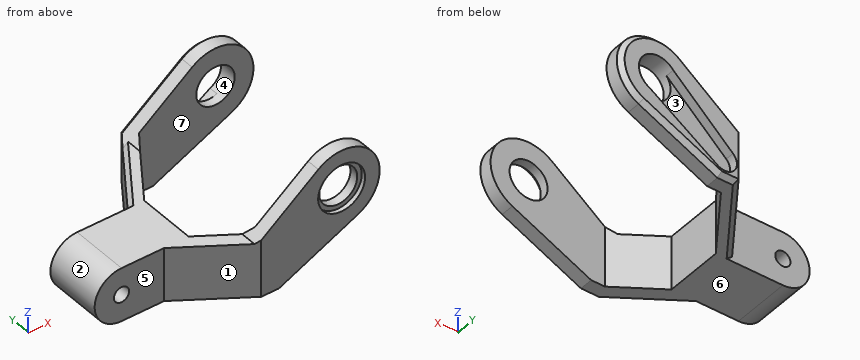
```python
from build123d import *

# Parameters (mm, degrees)
PAD012_DEPTH           = 10
CYLINDER024_R          = 4.3
CYLINDER024_DEPTH      = 14
CYLINDER024_ROLL_ANGLE = 90
CYLINDER017_R          = 4.25
CYLINDER017_DEPTH      = 10
CYLINDER016_R          = 5.25
CYLINDER016_DEPTH      = 10
FUSION009_ROLL_ANGLE   = 90
SKETCH005_R            = 1.7
PAD005_DEPTH           = 50
PAD006_DEPTH           = 40
CHAMFER004_SIZE        = 1


with BuildPart() as pad012:
    # Sketch012 → Pad012 (new body)
    with BuildSketch(Plane(origin=(0, 49, 0), x_dir=(-1, 0, 0), z_dir=(0, 1, 0))):
        with BuildLine():
            ThreePointArc((49.900014, 10.106834), (43.673915, 9.645687), (44.625156, 3.475427))
            Line((44.625156, 3.475427), (60.33289, -7.108383))
            ThreePointArc((60.33289, -7.108383), (64.021726, -6.539695), (63.746037, -2.817476))
            Line((49.900014, 10.106834), (63.746037, -2.817476))
        make_face()
    extrude(amount=PAD012_DEPTH)


with BuildPart() as fusion025:
    # Cylinder024 → Cylinder024 (new body)
    with BuildSketch(Plane.XY):
        Circle(CYLINDER024_R)
    extrude(amount=CYLINDER024_DEPTH)


with BuildPart() as fusion025_1:
    # Cylinder024 roll: moved
    add(fusion025.part.rotate(Axis((0, 0, 0), (1, 0, 0)), CYLINDER024_ROLL_ANGLE))


with BuildPart() as fusion025_2:
    # Cylinder024 placement: moved
    add(fusion025_1.part.moved(Location((-47, 58, 7))))

    # Fusion025: union Pad012
    add(pad012.part)


with BuildPart() as cylinder017:
    # Cylinder017 → Cylinder017 (new body)
    with BuildSketch(Plane.XY.offset(-5)):
        Circle(CYLINDER017_R)
    extrude(amount=CYLINDER017_DEPTH)


with BuildPart() as fusion009:
    # Cylinder016 → Cylinder016 (new body)
    with BuildSketch(Plane.XY):
        Circle(CYLINDER016_R)
    extrude(amount=CYLINDER016_DEPTH)

    # Fusion009: union Cylinder017
    add(cylinder017.part)


with BuildPart() as fusion009_1:
    # Fusion009 roll: moved
    add(fusion009.part.rotate(Axis((0, 0, 0), (1, 0, 0)), FUSION009_ROLL_ANGLE))


with BuildPart() as fusion009_2:
    # Fusion009 placement: moved
    add(fusion009_1.part.moved(Location((-47, 11, 7))))


with BuildPart() as pad005:
    # Sketch005 → Pad005 (new body)
    with BuildSketch(Plane(origin=(0, 55, 0), x_dir=(-1, 0, 0), z_dir=(0, 1, 0))):
        with BuildLine():
            ThreePointArc((52.215569, 13.711769), (39.756321, 11.447371), (43.374568, -0.688059))
            Line((43.374568, -0.688059), (61.000798, -9))
            Line((61.000798, -9), (89.000022, -9))
            ThreePointArc((89.000022, -9), (95, -3), (89.000022, 3))
            Line((66.000242, 3), (89.000022, 3))
            Line((52.215569, 13.711769), (66.000242, 3))
        make_face()
        with Locations((47, 7)):
            Circle(SKETCH005_R, mode=Mode.SUBTRACT)
        with Locations((89, -3)):
            Circle(SKETCH005_R, mode=Mode.SUBTRACT)
    extrude(amount=-PAD005_DEPTH)


with BuildPart() as cut036:
    # Sketch006 → Pad006 (new body)
    with BuildSketch(Plane.XY.offset(-20)):
        Polygon((-102.641426, 32.5), (-77.641426, 32.5), (-65, 51), (-36, 51), (-36, 47), (-64.091855, 47), (-74, 32.5), (-74, 19.5), (-64.091855, 13), (-36, 13), (-36, 10), (-65, 10), (-79.481134, 19.5), (-102.641426, 19.5), align=None)
    extrude(amount=PAD006_DEPTH)

    # Common: intersect Pad005
    add(pad005.part, mode=Mode.INTERSECT)

    # Chamfer004
    chamfer004_edges = [cut036.edges().sort_by_distance(p)[0] for p in [
        (-71.320713, 41.75, -9),
        (-71.820834, 41.018102, 3),
        (-63.000399, 51, -9),
        (-52.187683, 51, -4.844029),
        (-39.756321, 51, 11.447371),
    ]]
    chamfer(chamfer004_edges, length=CHAMFER004_SIZE)

    # Cut013: cut Fusion009
    add(fusion009_2.part, mode=Mode.SUBTRACT)

    # Cut036: cut Fusion025
    add(fusion025_2.part, mode=Mode.SUBTRACT)


solid = cut036.part
```
Geometry: final body of the model. Coordinates: model frame, mm. Face numbers are marked on the shaded views. A direction names the side the tool comes from. Give positions to 0.01 mm unless a question says otherwise; leave off trailing zeros. Write each loop counter-clockwise with the first axis right and the second up, starting at its lowest first coordinate (ties: lowest second). Pieces come first, ordered by that corner, then holes.
1. Section query B-B, the plane z = 6.25. Count the separate pieces of the cut face and the enclosed holes in it, then the cut area to 3 significant figures.
2. Reachability of the marked faces 5, 6 and 7 from +Z, -Z, +X, -X, +Y, -Y: full face, straight path, thin tool, end or side. Return the list, or none.
3. Pin query (flat end, axial travel): P1, Ø9.5, axis at y = 29, z = -5.5, coming from the +X side; P2, Ø5, axis at x = -80, y = 34, coming from the +Z side; P3, Ø5, axis at x = -54.5, y = 15, coming from the +Z side. Return the tip coordinate at first contact, or that it passes through.
4. Section query D-D, the plane z = -5.5. Return loops of the section in (x, y), then the cut area to 3 significant figures.
5. Section query A-A, the plane x = -53. Return loops of the section in (y, z).
6. Draft query along Z for the marked faces 1, 2, 3 and 4. Return one class per face: released by +Z, released by -Z, zero draft, split by the parting line, or undercut.
7. Line query: probe 1 along Z at (x, y) = (-89, 22); probe 2 along Y at (x, z) = (-56, -5); probe 3 along Y at (x, z) = (-84, 1). Output: solid intervals per line, ascending.
Computed:
1. separate pieces: 4
1. enclosed holes: 0
1. area: 95.1 mm2
2. face 5: +Z, -Z, -X, -Y
2. face 6: -Z, +X, -X, +Y, -Y
2. face 7: +Z, -Z, +X
3. P1: stops at x = -73.15
3. P2: stops at z = 3
3. P3: stops at z = 13.1
4. outline: (-94.45, 19.5) - (-79.48, 19.5) - (-65, 10) - (-53.58, 10) - (-53.58, 13) - (-64.09, 13) - (-74, 19.5) - (-74, 32.5) - (-64.09, 47) - (-53.58, 47) - (-53.58, 50) - (-55.92, 51) - (-57.95, 51) - (-57.95, 49) - (-64.54, 49) - (-64.54, 51) - (-65, 51) - (-77.64, 32.5) - (-94.45, 32.5) - close
4. area: 432 mm2
5. outline: (10, -5.23) - (13, -5.23) - (13, 13.1) - (10, 13.1) - close; (47, -5.23) - (50, -5.23) - (51, -4.12) - (51, -2.17) - (49, -2.17) - (49, 7.21) - (51, 7.21) - (51, 11.84) - (50, 13.1) - (47, 13.1) - close
6. face 1: zero draft
6. face 2: split by the parting line
6. face 3: undercut
6. face 4: undercut
7. probe 1: z = -9 to -4.7, -1.3 to 3
7. probe 2: y = 10 to 13, 47 to 51
7. probe 3: y = 19.5 to 32.5
